Can you work these out from the model? Positions are in its coordinate system, mm. A direction names the side the tool comes from. Give positions to 0.01 mm unless a question says otherwise; leave off trailing zeros. Loops run counter-clockwise (first coordinate to the right, second up) from the corner with the lowest first, then second, coordinate; pieces in that order, holes last. Notation, with made-up numbers: M -35.75,-33 L -16.75,-33 A11 cw -16.75,-27 Z; hole C 77.25,-26 d6. An arc over 180 degrees is marked long. Answer as a JSON object with one key per item and string values.
```python
from build123d import *

# Parameters (mm, degrees)
SKETCH4_R           = 25.817449465
CUT_EXTRUDE1_DEPTH  = 20
BOSS_EXTRUDE2_DEPTH = 6.5
BOSS_EXTRUDE3_DEPTH = 6.5
SKETCH7_R           = 2.75
BOSS_EXTRUDE4_DEPTH = 0.8
BOSS_EXTRUDE5_START = -0.8
SKETCH8_R           = 2.75
BOSS_EXTRUDE5_DEPTH = 0.8


with BuildPart() as part:
    # Sketch1 → Revolve1 (revolve)
    with BuildSketch(Plane.XY, mode=Mode.PRIVATE) as revolve1_sk:
        Polygon((-313.333333333, 0), (-313.333333333, 4), (-13.333333333, 4), (-13.333333333, 5), (6.666666667, 5), (6.666666667, 0), align=None)
    revolve(revolve1_sk.sketch.rotate(Axis((6.666666667, 0, 0), (-1, 0, 0)), 270), axis=Axis((6.666666667, 0, 0), (-1, 0, 0)))

    # Sketch2 → Revolve2 (revolve)
    with BuildSketch(Plane.XY, mode=Mode.PRIVATE) as revolve2_sk:
        Polygon((2.2, -4), (3.64, -4), (3.64, -13), (4.2, -16.175917819), (4.2, -24.824082181), (3.64, -28), (3.64, -95), (3.24, -95), (3.24, -195), (2.2, -195), align=None)
    revolve(revolve2_sk.sketch.rotate(Axis((2.2, -195, 0), (0, 1, 0)), 270), axis=Axis((2.2, -195, 0), (0, 1, 0)))

    # Sketch3 → Revolve3 (revolve)
    with BuildSketch(Plane.XY, mode=Mode.PRIVATE) as revolve3_sk:
        Polygon((-2.2, -195), (-3.24, -195), (-3.24, -95), (-3.64, -95), (-3.64, -35.5), (-4.2, -32.324082181), (-4.2, -23.675917819), (-3.64, -20.5), (-3.64, -4), (-2.2, -4), align=None)
    revolve(revolve3_sk.sketch.rotate(Axis((-2.2, -4, 0), (0, -1, 0)), 90), axis=Axis((-2.2, -4, 0), (0, -1, 0)))

    # Sketch4 → Cut-Extrude1 (cut)
    with BuildSketch(Plane(origin=(0, -190, 0), x_dir=(-1, 0, 0), z_dir=(0, 1, 0))):
        Circle(SKETCH4_R)
    extrude(amount=-CUT_EXTRUDE1_DEPTH, mode=Mode.SUBTRACT)

    # Sketch5 → Boss-Extrude2 (add)
    with BuildSketch(Plane(origin=(0, -190, 0), x_dir=(-1, 0, 0), z_dir=(0, 1, 0))):
        with BuildLine():
            ThreePointArc((-1.930000033, -2.250000045), (-1.18, 2e-09), (-1.930000036, 2.250000048))
            ThreePointArc((-1.930000036, 2.250000048), (-3.43000003, 3), (-4.93, 2.25))
            ThreePointArc((-4.93, 2.25), (-5.68, 0), (-4.93, -2.25))
            ThreePointArc((-4.93, -2.25), (-3.430000028, -3), (-1.930000033, -2.250000045))
        make_face()
    extrude(amount=-BOSS_EXTRUDE2_DEPTH)

    # Sketch6 → Boss-Extrude3 (add)
    with BuildSketch(Plane(origin=(0, -190, 0), x_dir=(-1, 0, 0), z_dir=(0, 1, 0))):
        with BuildLine():
            ThreePointArc((4.929999975, -2.250000034), (5.68, -2.1e-08), (4.93, 2.25))
            ThreePointArc((4.93, 2.25), (3.430000035, 3), (1.930000042, 2.250000056))
            ThreePointArc((1.930000042, 2.250000056), (1.18, 5e-09), (1.930000036, -2.250000048))
            ThreePointArc((1.930000036, -2.250000048), (3.430000009, -3), (4.929999975, -2.250000034))
        make_face()
    extrude(amount=-BOSS_EXTRUDE3_DEPTH)

    # Sketch7 → Boss-Extrude4 (add)
    with BuildSketch(Plane(origin=(1.18, 0, 0), x_dir=(0, 0, -1), z_dir=(1, 0, 0))):
        with BuildLine():
            Line((2.75, -196.339745962), (2.75, -190))
            Line((2.75, -190), (-2.75, -190))
            Line((-2.75, -190), (-2.75, -196.339745962))
            ThreePointArc((-2.75, -196.339745962), (-3.134679445, -199.715009665), (-4.268987342, -202.917154092))
            ThreePointArc((-4.268987342, -202.917154092), (0, -209.75), (4.268987342, -202.917154092))
            ThreePointArc((4.268987342, -202.917154092), (3.134679445, -199.715009665), (2.75, -196.339745962))
        make_face()
        with Locations((0, -205)):
            Circle(SKETCH7_R, mode=Mode.SUBTRACT)
    extrude(amount=BOSS_EXTRUDE4_DEPTH)

    # Sketch8 → Boss-Extrude5 (add)
    with BuildSketch(Plane(origin=(-1.18, 0, 0), x_dir=(0, 0, -1), z_dir=(1, 0, 0)).offset(BOSS_EXTRUDE5_START)):
        with BuildLine():
            Line((2.75, -196.339745962), (2.75, -190))
            Line((2.75, -190), (-2.75, -190))
            Line((-2.75, -190), (-2.75, -196.339745962))
            ThreePointArc((-2.75, -196.339745962), (-3.134679445, -199.715009665), (-4.268987342, -202.917154092))
            ThreePointArc((-4.268987342, -202.917154092), (0, -209.75), (4.268987342, -202.917154092))
            ThreePointArc((4.268987342, -202.917154092), (3.134679445, -199.715009665), (2.75, -196.339745962))
        make_face()
        with Locations((0, -205)):
            Circle(SKETCH8_R, mode=Mode.SUBTRACT)
    extrude(amount=BOSS_EXTRUDE5_DEPTH)


solid = part.part
```
1) For faces 1 (the flat face through (-313.333, 0, 0)), 2 (the cylindrical face through (-161.233, -3.905, -0.867)), 3 (the flat face through (-1.18, -200, 0)), which set-ups out of +Z, -Z, +X, -X, +Y, -Y let a thin tool reach every point of the face, with its end or its side?
Answer list:
{"face 1": "+Z, -Z, -X, +Y, -Y", "face 2": "-X", "face 3": "+Z, -Z, -Y"}
2) Suppose I cut it at B-B, the plane y = 0. Write out the boundary of the cut face in (x, z).
Answer list:
{"outline": "M -313.33,-4 L -13.33,-4 L -13.33,-5 L 6.67,-5 L 6.67,5 L -13.33,5 L -13.33,4 L -313.33,4 Z"}
3) Please list where these lines run through material, in increasing order: line 1 along Y through (x, z) = (1.3, 0); line 2 along X through (y, z) = (-94.5, -1); line 3 along Z through (x, y) = (-1.75, -205). Write a range as from..to.
Answer list:
{"line 1": "-209.75..-207.75, -202.25..5", "line 2": "-3.24..-1.16, 1.16..3.24", "line 3": "-4.75..-2.75, 2.75..4.75"}
4) Suppose I cut it at C-C, the plane x = -189.5. Write out the boundary of the cut face in (y, z), and give its area (3 significant figures).
Answer list:
{"outline": "C 0,0 d8", "area": "50.3 mm^2"}
5) Suppose I cut it at A-A, the plane y = -75. Write out the boundary of the cut face in (x, z), and give its area (3 significant figures).
Answer list:
{"outline": "C -2.2,0 d2.88; C 2.2,0 d2.88", "area": "13.0 mm^2"}
6) Will these pins go through, and if not, where does the flat tip stop? pin 1 Ø2 at (x, z) = (-197.5, 1.5) entering from -Y; pin 2 Ø2.5 at (x, z) = (3.5, 0.5) entering from +Y; pin 3 Ø0.9 at (x, z) = (2.5, 0.5) entering from -Y; pin 4 Ø5 at (y, z) = (-203, -1.5) entering from -X.
Answer list:
{"pin 1": "y = -3.97", "pin 2": "y = 5", "pin 3": "y = -196.5", "pin 4": "x = -1.98"}
7) If we mould it in two halves opening along X, with no side actions, what happens to faces 4 (the cylindrical face through (-1.59, -209.75, 0.13)), 5 (the flat face through (6.667, 0, 0)), 6 (the flat face through (1.18, -200, 0))? For each: +X half, -X half, draft (parallel to the pull), parting line (faces both ways), or undercut.
Answer list:
{"face 4": "draft", "face 5": "+X half", "face 6": "undercut"}
